from build123d import *

# Parameters (mm, degrees)
SKETCH1_R           = 7.5
SKETCH1_R_2         = 5
BOSS_EXTRUDE1_DEPTH = 2.75
SKETCH2_R           = 5
SKETCH2_R_2         = 3
BOSS_EXTRUDE2_DEPTH = 4
BOSS_EXTRUDE3_DEPTH = 2
FILLET1_R           = 2


with BuildPart() as part:
    # Sketch1 → Boss-Extrude1 (new, symmetric)
    with BuildSketch(Plane.XY):
        Circle(SKETCH1_R)
        Circle(SKETCH1_R_2, mode=Mode.SUBTRACT)
    extrude(amount=BOSS_EXTRUDE1_DEPTH, both=True)



with BuildPart() as body_2:
    # Sketch2 → Boss-Extrude2 (new, symmetric)
    with BuildSketch(Plane.XY):
        with Locations((0, 56)):
            Circle(SKETCH2_R)
        with Locations((0, 56)):
            Circle(SKETCH2_R_2, mode=Mode.SUBTRACT)
    extrude(amount=BOSS_EXTRUDE2_DEPTH, both=True)


with BuildPart() as part_1:
    add(part.part)

    add(body_2.part)  # Boss-Extrude3 merges body 2
    # Sketch3 → Boss-Extrude3 (add, symmetric)
    with BuildSketch(Plane.XY):
        with BuildLine():
            Line((-3.043800059, 52.033227861), (-3.543272067, 6.610236233))
            ThreePointArc((-3.543272067, 6.610236233), (0, 7.5), (3.543272067, 6.610236233))
            Line((3.543272067, 6.610236233), (3.043800059, 52.033227861))
            ThreePointArc((3.043800059, 52.033227861), (0, 51), (-3.043800059, 52.033227861))
        make_face()
    extrude(amount=BOSS_EXTRUDE3_DEPTH, both=True)

    # Fillet1
    fillet1_edges = [part_1.edges().sort_by_distance(p)[0] for p in [
        (3.043800059, 52.033227861, 0),
        (-3.043800059, 52.033227861, 0),
        (-3.543272067, 6.610236233, 0),
        (3.543272067, 6.610236233, 0),
    ]]
    fillet(fillet1_edges, radius=FILLET1_R)


solid = part_1.part
Read the model definition and answer for the solid it produces. Units are mm, in the model's axes. A direction names the side the tool comes from. Round coordinates to 2 decimals unless told otherwise and drop trailing zeros. Write each loop counter-clockwise with the first axis right and the second up, starting at its lowest first coordinate (ties: lowest second). Pieces come first, ordered by that corner, then holes.
Q1. The mould has two halves that part along X. Classify faces 6 (the face through (0, 59, 0)), 7 (the face through (-1.63, -7.32, 0.04)), 8 (the face through (3.3, 56.1, -4)), 9 (the face through (3.75, 6.81, 0.03)): released by +X, released by -X, zero draft, split by the parting line, or undercut.
Values:
face 6: undercut
face 7: split by the parting line
face 8: zero draft
face 9: released by +X
Q2. Straight lines are drawn through the part: line 1 (Y direction, x = 0, z = -0.75); line 2 (Y direction, x = 0, z = 2.25); line 3 (Y direction, x = -2.75, z = 1). For each, find the intervals that lie inside material, in ascending order.
Values:
line 1: y = -7.5 to -5, 5 to 53, 59 to 61
line 2: y = -7.5 to -5, 5 to 7.5, 51 to 53, 59 to 61
line 3: y = -6.98 to -4.18, 4.18 to 54.8, 57.2 to 60.18
Q3. Find section A-A on x = 0. Determine the outline of the cut face in (y, z).
Values:
outline: (-7.5, -2.75) - (-5, -2.75) - (-5, 2.75) - (-7.5, 2.75) - close; (5, -2.75) - (7.5, -2.75) - (7.5, -2) - (51, -2) - (51, -4) - (53, -4) - (53, 4) - (51, 4) - (51, 2) - (7.5, 2) - (7.5, 2.75) - (5, 2.75) - close; (59, -4) - (61, -4) - (61, 4) - (59, 4) - close
Q4. A tool of negligible diameter and unlimited length cuts with its end or side. For faces 1 (the face through (3.198, 51.902, -0.028)), 2 (the face through (2, -5, 2.75)), 3 (the face through (2, -5, -2.75)), 4 (the face through (-3.198, 51.902, -0.028)), 5 (the face through (3.3, 56.1, 4)), from which of +Z, -Z, +X, -X, +Y, -Y can it reach the whole face along a straight path? Write none if from no direction.
Values:
face 1: +Z, -Z, +X
face 2: +Z, +X, -X, -Y
face 3: -Z, +X, -X, -Y
face 4: +Z, -Z, -X
face 5: +Z, +X, -X, +Y, -Y
Q5. Find section D-D on y = 56. Determine the outline of the cut face in (x, z).
Values:
outline: (-5, -4) - (-3, -4) - (-3, 4) - (-5, 4) - close; (3, -4) - (5, -4) - (5, 4) - (3, 4) - close
Q6. Find section C-C on z = -0.5. Determine the outline of the cut face in (x, y).
Values:
outline: (-4.37, 6.1) arc R7.5 ccw (long way) to (4.37, 6.1) arc R2 cw to (3.53, 7.7) - (3.05, 51.13) arc R2 cw to (3.61, 52.54) arc R5 ccw (long way) to (-3.61, 52.54) arc R2 cw to (-3.05, 51.13) - (-3.53, 7.7) arc R2 cw to start; hole circle Ø10 at (0, 0); hole circle Ø6 at (0, 56)
Q7. Find section B-B on y = 0. Determine the outline of the cut face in (x, z), and give its area (3 significant figures).
Values:
outline: (-7.5, -2.75) - (-5, -2.75) - (-5, 2.75) - (-7.5, 2.75) - close; (5, -2.75) - (7.5, -2.75) - (7.5, 2.75) - (5, 2.75) - close
area: 27.5 mm2
Q8. Flat-ended cylindrical pins translate along their axes: P1, Ø7, axis at x = 1.5, y = 24.5, coming from the -Z side; P2, Ø4, axis at y = 50.5, z = 1.5, coming from the -X side; P3, Ø1.5, axis at y = 54, z = 1, coming from the +X side; P4, Ø2, axis at x = -0.5, z = -3, coming from the +Y side. Find the tip coordinate at first contact, or state that the pin passes through.
Values:
P1: stops at z = -2
P2: stops at x = -3.57
P3: stops at x = 4.84
P4: stops at y = 61
